Drawing for the job (mm, zero at the part's lowest x, y, z). A direction names the side the tool comes from. Round coordinates to 2 decimals unless told otherwise and drop trailing zeros. Order: outer loops, then holes, each group sorted by start corner. A loop starts at its lowest first (then second) coordinate and runs counter-clockwise, first axis right, second up. Notation, with made-up numbers: (2.25, 43.25) -> (31.25, 43.25) arc R26 cw to (31.25, 77.25) -> close; hole circle Ø8 at (41, 6.25). An arc over 180 degrees is marked (long way). Use CSV: the item, a comma, the result in double quotes.
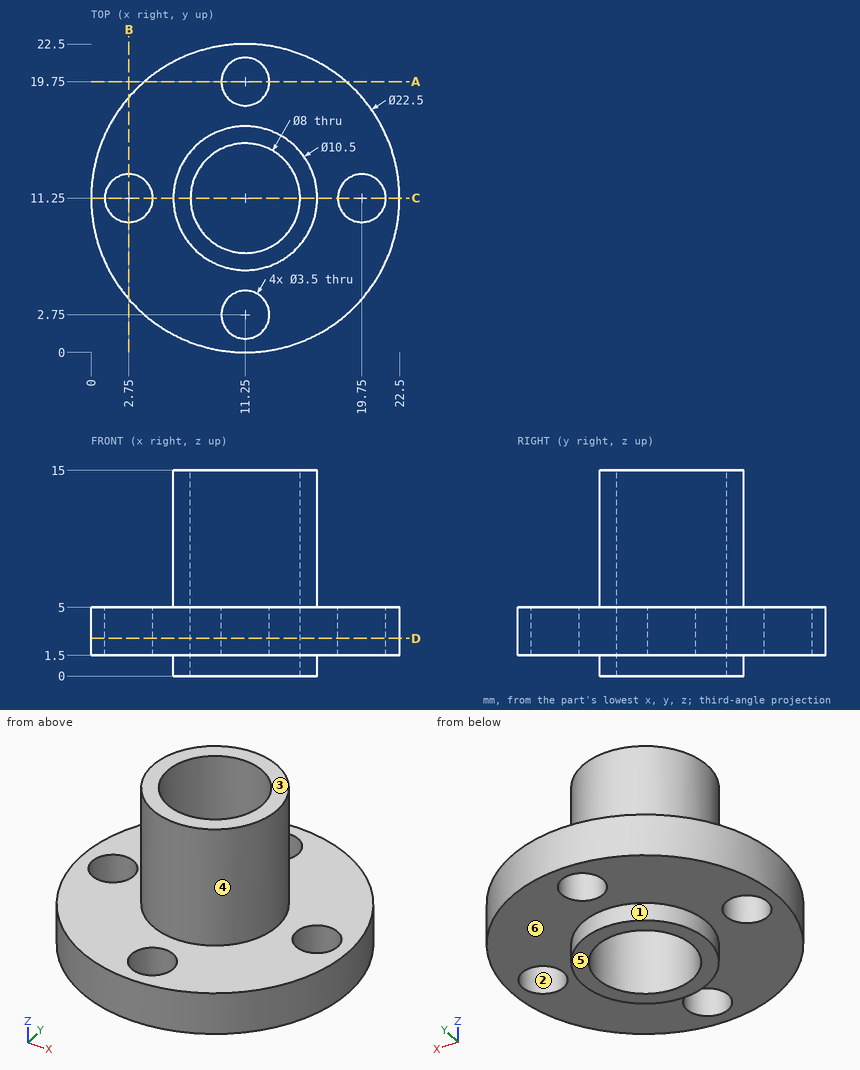
Q1. Which spindle directions (+Z, -Z, +X, -X, +Y, -Y) get a long thin tool onto all of the face, cutting with end or side? Do the marked faces 4, 5 and 6. Say none if no direction does.
From the geometry:
face 4,"+Z"
face 5,"-Z, +X, -X, +Y, -Y"
face 6,"-Z"
Q2. Cut at C-C (y = 11.25). Give the cut face in (x, z), plus the area to 3 significant figures.
From the geometry:
outline,"(0, 1.5) -> (1, 1.5) -> (1, 5) -> (0, 5) -> close; (4.5, 1.5) -> (6, 1.5) -> (6, 0) -> (7.25, 0) -> (7.25, 15) -> (6, 15) -> (6, 5) -> (4.5, 5) -> close; (15.25, 0) -> (16.5, 0) -> (16.5, 1.5) -> (18, 1.5) -> (18, 5) -> (16.5, 5) -> (16.5, 15) -> (15.25, 15) -> close; (21.5, 1.5) -> (22.5, 1.5) -> (22.5, 5) -> (21.5, 5) -> close"
area,"55.0 mm²"
Q3. Mould opens along Y. For the marked faces 1, 2 and 3 say: +Y half, -Y half, draft (parallel to the pull), parting line (faces both ways), or undercut.
From the geometry:
face 1,"parting line"
face 2,"undercut"
face 3,"draft"
Q4. Pin check, flat tips, straight feed: pin 1 (2 mm diameter, centred on x = 19.5, y = 3, fed in from -Z); pin 2 (7 mm diameter, centred on x = 11.25, y = 11.25, fed in from +Z); pin 3 (1.5 mm diameter, centred on y = 12.5, z = 6.5, fed in from +X). Stop position of each tip, or through.
From the geometry:
pin 1,"stops at z = 1.5"
pin 2,"passes through"
pin 3,"stops at x = 16.48"
Q5. Cut at D-D (z = 2.75). Give the cut face in (x, y), plus the area to 3 significant figures.
From the geometry:
outline,"circle Ø22.5 at (11.25, 11.25); hole circle Ø3.5 at (2.75, 11.25); hole circle Ø8 at (11.25, 11.25); hole circle Ø3.5 at (11.25, 2.75); hole circle Ø3.5 at (11.25, 19.75); hole circle Ø3.5 at (19.75, 11.25)"
area,"309 mm²"
Q6. Probe line 1 along X through (y, z) = (10.5, 4.75); line 2 along Z through (x, y) = (20.75, 6.5); line 3 along Y through (x, z) = (2.75, 4). List the from-to ranges inside material, lowest first.
From the geometry:
line 1,"x = 0.03 to 1.17, 4.33 to 7.32, 15.18 to 18.17, 21.33 to 22.47"
line 2,"z = 1.5 to 5"
line 3,"y = 3.88 to 9.5, 13 to 18.62"
Q7. Cut at A-A (y = 19.75). Give the cut face in (x, z), plus the area to 3 significant figures.
From the geometry:
outline,"(3.88, 1.5) -> (9.5, 1.5) -> (9.5, 5) -> (3.88, 5) -> close; (13, 1.5) -> (18.62, 1.5) -> (18.62, 5) -> (13, 5) -> close"
area,"39.3 mm²"
